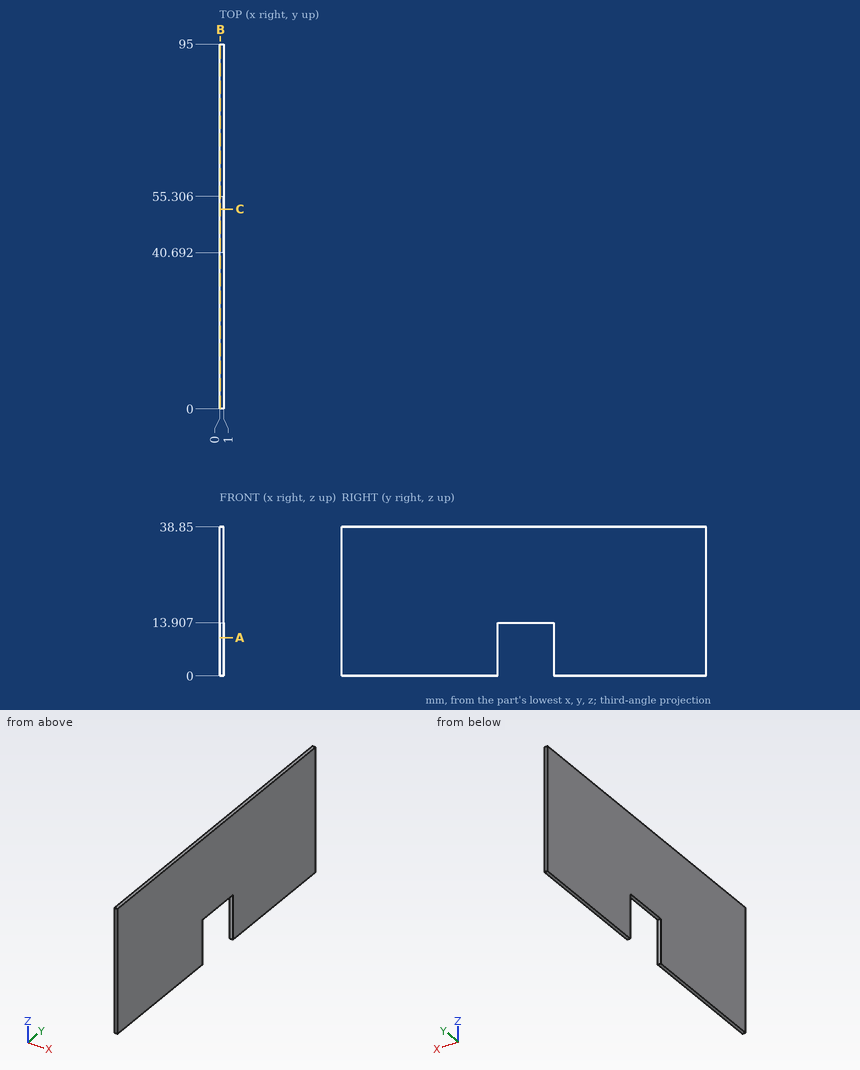
Geometry check sheet. Reference: drawing and pictorial views, mm from the part's lowest x, y, z. Coordinates: 2 decimals unless noted, no trailing zeros. Write each loop counter-clockwise with the first axis right and the second up, starting at its lowest first coordinate (ties: lowest second). Pieces come first, ordered by that corner, then holes. Notation, with made-up numbers: M -12.75,-7.5 L 34.25,-7.5 A20 cw 34.25,-2.5 Z; hole C -19,79.25 d3. An arc over 180 degrees is marked long. Use one line per item in the form item = value.
Item 1: Sectioned sample at A-A, the plane z = 10. Record the cut outline in (x, y).
Answer below:
outline = M 0,0 L 1,0 L 1,40.69 L 0,40.69 Z; M 0,55.31 L 1,55.31 L 1,95 L 0,95 Z
Item 2: Sectioned sample at B-B, the plane x = 0.15. Record the cut outline in (y, z), and give its area (3 significant figures).
Answer below:
outline = M 0,0 L 40.69,0 L 40.69,13.91 L 55.31,13.91 L 55.31,0 L 95,0 L 95,38.85 L 0,38.85 Z
area = 3,490 mm^2
Item 3: Gauge pin test, flat end, axial feed: pin 1 Ø0.5 at (x, y) = (0.5, 51.5) entering from -Z. Record the tip position at first contact, or that the pin passes through.
Answer below:
pin_1 = 13.91
Item 4: Material ranges on L1, parallel to Y at x = 0.95, z = 6.5, recorded low to high. Write a range as from..to.
Answer below:
L1 = 0..40.69, 55.31..95
Item 5: Sectioned sample at C-C, the plane y = 52. Record the cut outline in (x, z).
Answer below:
outline = M 0,13.91 L 1,13.91 L 1,38.85 L 0,38.85 Z
